from build123d import *

# Parameters (mm, degrees)
SKETCH_1_W          = 29
SKETCH_1_H          = 29
EXTRUDE_1_DEPTH     = 1
SKETCH_2_W          = 31
SKETCH_2_H          = 31
SKETCH_2_W_2        = 29
SKETCH_2_H_2        = 29
EXTRUDE_2_DEPTH     = 13
EXTRUDE_4_DEPTH     = 5
CUT_EXTRUDE_START   = -14
CUT_EXTRUDE_2_DEPTH = 27
SKETCH_5_R          = 2.15366908
EXTRUDE_5_DEPTH     = 1
FILLET_2_R          = 2
FILLET_3_R          = 1.5
SKETCH_6_R          = 1.5
CUT_EXTRUDE_3_DEPTH = 10


with BuildPart() as part:
    # 草图1 → 凸台-拉伸1 (new body)
    with BuildSketch(Plane.XY):
        Rectangle(SKETCH_1_W, SKETCH_1_H)
        Polygon((-11.5, 0), (-11.5, 9.5), (11.5, 9.5), (11.5, -5.5), (-11.5, -5.5), align=None, mode=Mode.SUBTRACT)
    extrude(amount=EXTRUDE_1_DEPTH)

    # 草图2 → 凸台-拉伸2 (add)
    with BuildSketch(Plane.XY.offset(1)):
        Rectangle(SKETCH_2_W, SKETCH_2_H)
        Rectangle(SKETCH_2_W_2, SKETCH_2_H_2, mode=Mode.SUBTRACT)
    extrude(amount=-EXTRUDE_2_DEPTH)

    # 草图3 → 凸台-拉伸4 (add)
    with BuildSketch(Plane(origin=(15.5, 0, 0), x_dir=(0, 0, -1), z_dir=(1, 0, 0))):
        with BuildLine():
            Line((1.684082639, 8.989995997), (0.397094894, -5.595641246))
            Line((0.397094894, -5.595641246), (10.451208148, -10.79214922))
            Line((10.451208148, -10.79214922), (9.295909354, 8.989995997))
            ThreePointArc((9.295909354, 8.989995997), (5.489995997, 12.795909354), (1.684082639, 8.989995997))
        make_face()
    extrude_4 = extrude(amount=EXTRUDE_4_DEPTH)

    # 草图4 → 切除-拉伸2 (cut)
    with BuildSketch(Plane(origin=(0, -0.077997079, -0.883953322), x_dir=(1, 0, 0), z_dir=(0, 0.08789514896151537, 0.9961297319069606)).offset(CUT_EXTRUDE_START)):
        Polygon((18, 9.103224997), (20.5, -9.831770213), (20.5, 13.243659675), (18, 13.243659675), align=None)
    cut_extrude_2 = extrude(amount=CUT_EXTRUDE_2_DEPTH, mode=Mode.SUBTRACT)

    # 草图5 → 凸台-拉伸5 (add)
    with BuildSketch(Plane(origin=(18, 0, 0), x_dir=(0, 0, -1), z_dir=(1, 0, 0))):
        with Locations(Location((5.489995997, 8.989995997, 0), (0, 0, 183.893189549))):
            Circle(SKETCH_5_R)
    extrude_5 = extrude(amount=EXTRUDE_5_DEPTH)

    # 镜向1: 凸台-拉伸4, 切除-拉伸2, 凸台-拉伸5 across plane
    add(extrude_4.mirror(Plane(origin=(0, 0, 0), x_dir=(0, 0, 1), z_dir=(1, 0, 0))))
    add(cut_extrude_2.mirror(Plane(origin=(0, 0, 0), x_dir=(0, 0, 1), z_dir=(1, 0, 0))), mode=Mode.SUBTRACT)
    add(extrude_5.mirror(Plane(origin=(0, 0, 0), x_dir=(0, 0, 1), z_dir=(1, 0, 0))))

    # 圆角2
    fillet_2_edges = [part.edges().sort_by_distance(p)[0] for p in [
        (15.5, -15.5, -5.5),
        (-15.5, -15.5, -5.5),
        (-15.5, 15.5, -5.5),
        (15.5, 15.5, -5.5),
    ]]
    fillet(fillet_2_edges, radius=FILLET_2_R)

    # 圆角3
    fillet_3_edges = [part.edges().sort_by_distance(p)[0] for p in [
        (-18, -10.79214922, -10.451208148),
        (-17.716616755, -5.595641246, -0.397094894),
        (18, -10.79214922, -10.451208148),
        (17.716616755, -5.595641246, -0.397094894),
    ]]
    fillet(fillet_3_edges, radius=FILLET_3_R)

    # 草图6 → 切除-拉伸3 (cut)
    with BuildSketch(Plane(origin=(0, -14.5, 0), x_dir=(1, 0, 0), z_dir=(0, 1, 0))):
        with Locations(Location((0, 8.292466775, 0), (0, 0, 270))):
            Circle(SKETCH_6_R)
    extrude(amount=-CUT_EXTRUDE_3_DEPTH, mode=Mode.SUBTRACT)


solid = part.part
Build history of the part. All positions in model axes, mm. A direction names the side the tool comes from. Round coordinates to 2 decimals unless told otherwise and drop trailing zeros. Order: outer loops, then holes, each group sorted by start corner. A loop starts at its lowest first (then second) coordinate and runs counter-clockwise, first axis right, second up. Notation, with made-up numbers: M -29.5,-19 L 21.5,-19 A26 ccw 21.5,13 Z; hole C 17.25,40 d5. An arc over 180 degrees is marked long. Use CSV: the item, a comma, the result in double quotes. Start each with the question number.
(1) Tool access for faces 1 (the face through (17.278, 0.293, -9.804)), 2 (the face through (11.5, 2.1, 0.5)), 3 (the face through (-16.732, 12.795, -5.574)): list every direction of +Z, -Z, +X, -X, +Y, -Y with a clear straight run to the whole face (end or side of a thin tool).
(2) Flat gauge pins, fed straight in: P1, Ø1.5, axis at y = -1.5, z = -6.5, coming from the +X side; P2, Ø6, axis at y = 0.5, z = -5.5, coming from the -X side; P3, Ø6.5, axis at y = -5.5, z = -6.5, coming from the -X side; P4, Ø3, axis at y = -10.5, z = -8.5, coming from the -X side. Where does each tip first touch, or does it go through?
(3) Cut at B-B on z = -11. List the corners of the cut face in (x, y).
(4) Cut at C-C on y = -13. List the corners of the cut face in (x, z), then the cut area to 3 significant figures.
(5) Drill centre lines: probe 1 along Y at (x, z) = (-2, -10.75); probe 2 along X at (y, z) = (-5, -4.5). Where is each one in solid material? Low to high.
(6) Mould opens along X. For faces 4 (the face through (0, -7, 1)), 5 (the face through (18, 12, -6)), 6 (the face through (-0.2, 9.5, 0.5)) say: +X half, -X half, draft (parallel to the pull), parting line (faces both ways), or undercut.
(7) Cut at D-D on y = -4. List the corners of the cut face in (x, z), then the cut area to 3 significant figures.
(8) Cut at A-A on x = 0. List the corners of the cut face in (y, z), then the cut area to 3 significant figures.
Findings:
1,face 1,"-Z, +X, +Y"
1,face 2,"+Z, -Z"
1,face 3,"-X, +Y"
2,P1,"stops at x = 19.42"
2,P2,"stops at x = -19.47"
2,P3,"stops at x = -20.28"
2,P4,"stops at x = -20.38"
3,outline,"M -15.5,-13.5 A2 ccw -13.5,-15.5 L 13.5,-15.5 A2 ccw 15.5,-13.5 L 15.5,13.5 A2 ccw 13.5,15.5 L -13.5,15.5 A2 ccw -15.5,13.5 Z; hole M -14.5,-14.5 L 14.5,-14.5 L 14.5,14.5 L -14.5,14.5 Z"
4,outline,"M -15.5,-12 L -14.5,-12 L -14.5,0 L 14.5,0 L 14.5,-12 L 15.5,-12 L 15.5,1 L -15.5,1 Z"
4,area,"55.0 mm^2"
5,probe 1,"y = -15.5 to -14.5, 14.5 to 15.5"
5,probe 2,"x = -19.81 to -14.5, 14.5 to 19.81"
6,face 4,"draft"
6,face 5,"+X half"
6,face 6,"undercut"
7,outline,"M -19.72,-0.54 L -19.61,-10.05 L -15.5,-10.05 L -15.5,-12 L -14.5,-12 L -14.5,0 L -11.5,0 L -11.5,1 L -15.5,1 L -15.5,-0.54 Z; M 11.5,0 L 14.5,0 L 14.5,-12 L 15.5,-12 L 15.5,-10.05 L 19.61,-10.05 L 19.72,-0.54 L 15.5,-0.54 L 15.5,1 L 11.5,1 Z"
7,area,"111 mm^2"
8,outline,"M -15.5,-12 L -14.5,-12 L -14.5,-9.79 L -15.5,-9.79 Z; M -15.5,-6.79 L -14.5,-6.79 L -14.5,0 L -5.5,0 L -5.5,1 L -15.5,1 Z; M 9.5,0 L 14.5,0 L 14.5,-12 L 15.5,-12 L 15.5,1 L 9.5,1 Z"
8,area,"37.0 mm^2"
